from build123d import *

# Parameters (mm, degrees)
SKETCH1_W           = 54
SKETCH1_H           = 50
SKETCH1_W_2         = 48
SKETCH1_H_2         = 6
BOSS_EXTRUDE1_DEPTH = 3
SKETCH2_W           = 2
SKETCH2_H           = 3
SKETCH2_W_2         = 1.834512626
SKETCH2_H_2         = 2.85876986
BOSS_EXTRUDE2_DEPTH = 10


with BuildPart() as part:
    # Sketch1 → Boss-Extrude1 (new body)
    with BuildSketch(Plane.XY):
        with Locations((27, 25)):
            Rectangle(SKETCH1_W, SKETCH1_H)
        with Locations((27, 25)):
            Rectangle(SKETCH1_W_2, SKETCH1_H_2, mode=Mode.SUBTRACT)
    extrude(amount=BOSS_EXTRUDE1_DEPTH)

    # Sketch2 → Boss-Extrude2 (add)
    with BuildSketch(Plane(origin=(0, 0, 0), x_dir=(-1, 0, 0), z_dir=(0, 0, -1))):
        with Locations((-40, 44.5)):
            Rectangle(SKETCH2_W, SKETCH2_H)
        with Locations((-14, 44.5)):
            Rectangle(SKETCH2_W, SKETCH2_H)
        with Locations((-40.082743687, 5.57061507)):
            Rectangle(SKETCH2_W_2, SKETCH2_H_2)
        with Locations((-14, 5.5)):
            Rectangle(SKETCH2_W, SKETCH2_H)
    extrude(amount=BOSS_EXTRUDE2_DEPTH)


solid = part.part
Design review of the part built by this model. Coordinates are the model's own, in mm. A direction names the side the tool comes from. Round coordinates to 2 decimals unless told otherwise and drop trailing zeros. Order: outer loops, then holes, each group sorted by start corner. A loop starts at its lowest first (then second) coordinate and runs counter-clockwise, first axis right, second up.
1) Consider section D-D (y = 8). State the section outline as (x, z) points, plus the area to 3 significant figures.
The answers:
outline: (0, 0) - (54, 0) - (54, 3) - (0, 3) - close
area: 162 mm2
2) For L1, parallel to Y at x = 32.5, z = 2.5; L2, parallel to X at y = 6.5, z = -1; L3, parallel to X at y = 45.5, z = -3, list the stretches that pass through material, from the lowest coordinate up.
The answers:
L1: y = 0 to 22, 28 to 50
L2: x = 13 to 15, 39.17 to 41
L3: x = 13 to 15, 39 to 41
3) Consider section C-C (x = 29.5). State the section outline as (y, z) points, plus the area to 3 significant figures.
The answers:
outline: (0, 0) - (22, 0) - (22, 3) - (0, 3) - close; (28, 0) - (50, 0) - (50, 3) - (28, 3) - close
area: 132 mm2
4) Consider section B-B (y = 25.5). State the section outline as (x, z) points.
The answers:
outline: (0, 0) - (3, 0) - (3, 3) - (0, 3) - close; (51, 0) - (54, 0) - (54, 3) - (51, 3) - close
5) Draft analysis for pull direction X (two halves, no side actions). For faces 5 (the flat face through (54, 25, 1)), 6 (the flat face through (14, 6, -10)), 7 (the flat face through (27, 28, 1)), state which applies: released by +X, released by -X, zero draft, split by the parting line, or undercut.
The answers:
face 5: released by +X
face 6: zero draft
face 7: undercut
6) Clearance check with flat-ended pins moving along their axes: pin 1 Ø0.9 at (y, z) = (6, -5.5) entering from +X; pin 2 Ø1.6 at (x, z) = (14.5, -3.5) entering from -Y; pin 3 Ø2 at (x, z) = (40.5, -3.5) entering from +Y. State where each tip first meets the part, or that it passes through.
The answers:
pin 1: stops at x = 41
pin 2: stops at y = 4
pin 3: stops at y = 46
7) Machinability: for faces 1 (the flat face through (39, 44, -5)), 2 (the flat face through (40, 4.141, -5)), 3 (the flat face through (41, 44, -5)), 4 (the flat face through (14, 43, -5)), which of the approach directions +Z, -Z, +X, -X, +Y, -Y give a long, thin tool a straight path to every point of the face, cutting with its end or side? Answer none if there is none.
The answers:
face 1: -Z, +Y, -Y
face 2: -Z, +X, -Y
face 3: -Z, +X, +Y, -Y
face 4: -Z, +X, -X
8) Consider section A-A (z = -1). State the section outline as (x, y) points, plus the area to 3 significant figures.
The answers:
outline: (13, 4) - (15, 4) - (15, 7) - (13, 7) - close; (13, 43) - (15, 43) - (15, 46) - (13, 46) - close; (39, 43) - (41, 43) - (41, 46) - (39, 46) - close; (39.17, 4.14) - (41, 4.14) - (41, 7) - (39.17, 7) - close
area: 23.2 mm2
